Design review of the part built by this model. Coordinates are the model's own, in mm. A direction names the side the tool comes from. Round coordinates to 2 decimals unless told otherwise and drop trailing zeros. Order: outer loops, then holes, each group sorted by start corner. A loop starts at its lowest first (then second) coordinate and runs counter-clockwise, first axis right, second up. Notation, with made-up numbers: (13, -11.75) - (67, -11.75) arc R20 ccw to (67, 8.25) - close; hole circle Ø6 at (75, -30). An arc over 180 degrees is marked (long way). Write item = value, one per line.
from build123d import *

# Parameters (mm, degrees)
F0_W     = 76.2
F0_H     = 76.2
F1_DEPTH = 25.4
F0_W_2   = 86.104107
F0_H_2   = 86.104107
F2_DEPTH = 12.7


with BuildPart() as f1:
    # F0 (on Front) → F1 (new body)
    with BuildSketch(Plane.XZ):
        with Locations((-6.351506, 13.068704)):
            Rectangle(F0_W, F0_H)
    extrude(amount=F1_DEPTH)

    # F0 (on Front) → F2 (join)
    with BuildSketch(Plane.XZ):
        with Locations((-6.351506, 13.068703)):
            Rectangle(F0_W_2, F0_H_2)
        with Locations((-6.351506, 13.068704)):
            Rectangle(F0_W, F0_H, mode=Mode.SUBTRACT)
    extrude(amount=F2_DEPTH)


solid = f1.part
Item 1: Take a section at C-C, the plane y = -20. State the section outline as (x, z) points, and give its area (3 significant figures).
Data:
outline = (-44.45, -25.03) - (31.75, -25.03) - (31.75, 51.17) - (-44.45, 51.17) - close
area = 5,810 mm2
Item 2: Take a section at B-B, the plane x = 28. State the section outline as (y, z) points, and give its area (3 significant figures).
Data:
outline = (-25.4, -25.03) - (-12.7, -25.03) - (-12.7, -29.98) - (0, -29.98) - (0, 56.12) - (-12.7, 56.12) - (-12.7, 51.17) - (-25.4, 51.17) - close
area = 2,060 mm2
Item 3: For line 1 along X through (y, z) = (-23.25, -13); line 2 along Z through (x, y) = (3, -21.5), list the stretches that pass through material, from the lowest coordinate up. Write a range as [from, to].
Data:
line_1 = [-44.45, 31.75]
line_2 = [-25.03, 51.17]
Item 4: Take a section at A-A, the plane z = -6. State the section outline as (x, y) points.
Data:
outline = (-49.4, -12.7) - (-44.45, -12.7) - (-44.45, -25.4) - (31.75, -25.4) - (31.75, -12.7) - (36.7, -12.7) - (36.7, 0) - (-49.4, 0) - close
Item 5: Insertion check: P1, Ø10, axis at x = -17, y = -14.5, coming from the -Z side; P2, Ø6, axis at x = 22.5, y = -21, coming from the -Z side; P3, Ø4, axis at y = -19.5, z = 9, coming from the +X side; P4, Ø6.5, axis at y = -19, z = 12, coming from the -X side. Each pin has a flat end and moves straight along its axis. Give the tip position at first contact, or say it passes through.
Data:
P1 = -29.98
P2 = -25.03
P3 = 31.75
P4 = -44.45
Item 6: For faces 1 (the face through (-7, -19, 51.169)), 2 (the face through (31.748, -19, 13)), 3 (the face through (-44.452, -19, 13)), 4 (the face through (-7, -19, -25.031)), list the 3-axis set-ups (+Z, -Z, +X, -X, +Y, -Y) from which the entire face can be reached by the end or side of a thin tool; tool diameter is ignored.
Data:
face_1 = +Z, +X, -X, -Y
face_2 = +Z, -Z, +X, -Y
face_3 = +Z, -Z, -X, -Y
face_4 = -Z, +X, -X, -Y
